Model file for the job. Use its own axes, mm. Face numbers are marked on the shaded views. A direction names the side the tool comes from. Coordinates: 2 decimals unless noted, no trailing zeros. Write each loop counter-clockwise with the first axis right and the second up, starting at its lowest first coordinate (ties: lowest second). Pieces come first, ordered by that corner, then holes.
Q1. Which spindle directions (+Z, -Z, +X, -X, +Y, -Y) get a long thin tool onto all of the face, cutting with end or side? Do the marked faces 4, 5 and 6. Say none if no direction does.
Q2. Drill centre lines: probe 1 along Y at (x, z) = (7.5, 0) (3 decimals); probe 2 along X at (y, z) = (0.5, -3.75); probe 3 along X at (y, z) = (-4.75, -1.5). Where is each one in solid material? Low to high.
Q3. Pull direction Y, two halves, no side cores. Call the marked faces 1, 2 and 3: released by +Y, released by -Y, zero draft, split by the parting line, or undercut.
Q4. Pin check, flat tips, straight feed: P1, Ø1, axis at y = 0, z = 1, coming from the -X side; P2, Ø2, axis at x = -5, z = 4, coming from the -Y side; P3, Ø1.5, axis at x = -5.5, y = 0.5, coming from the +Z side; P4, Ø4, axis at x = 1.5, y = -2.5, coming from the -Z side. Stop position of each tip, or through.
Q5. Band-saw the part on C-C, the plane x = 4. Write the cut outline in (y, z) (3 decimals), plus the area to 3 significant figures.
Q6. Band-saw the part on B-B, the plane x = 0.5. Write the cut outline in (y, z) (1 decimal).
from build123d import *

# Parameters (mm, degrees)
F0_W     = 11.1125
F0_H     = 3.175
F5_DEPTH = 3.175
F6_SIZE  = 0.254
F7_SIZE  = 0.508


with BuildPart() as f1:
    # F0 (on Front) → F1 (revolve)
    with BuildSketch(Plane.XZ):
        Polygon((-1.5875, 0), (-1.5875, 4.7625), (-1.5875, 5.55625), (-7.14375, 5.55625), (-7.14375, 0), align=None)
    revolve(axis=Axis((2.778125, 0, 0), (1, 0, 0)))

    # F0 (on Front) → F2 (revolve)
    with BuildSketch(Plane.XZ):
        Polygon((1.5875, 3.175), (1.5875, 4.7625), (-1.5875, 4.7625), (-1.5875, 0), (1.5875, 0), align=None)
    revolve(axis=Axis((2.778125, 0, 0), (1, 0, 0)))

    # F0 (on Front) → F3 (revolve)
    with BuildSketch(Plane.XZ):
        with Locations((7.14375, 1.5875)):
            Rectangle(F0_W, F0_H)
    revolve(axis=Axis((2.778125, 0, 0), (1, 0, 0)))

    # F4 (on face) → F5 (cut)
    with BuildSketch(Plane(origin=(-7.14375, 0, 0), x_dir=(0, -1, 0), z_dir=(-1, 0, 0))):
        Polygon((1.833087, 0), (0.916544, 1.5875), (-0.916544, 1.5875), (-1.833087, 0), (-0.916544, -1.5875), (0.916544, -1.5875), align=None)
    extrude(amount=-F5_DEPTH, mode=Mode.SUBTRACT)

    # F6
    f6_edges = [f1.edges().sort_by_distance(p)[0] for p in [
        (-7.14375, 0, -5.55625),
    ]]
    chamfer(f6_edges, length=F6_SIZE)

    # F7
    f7_edges = [f1.edges().sort_by_distance(p)[0] for p in [
        (12.7, 0, -3.175),
    ]]
    chamfer(f7_edges, length=F7_SIZE)


solid = f1.part
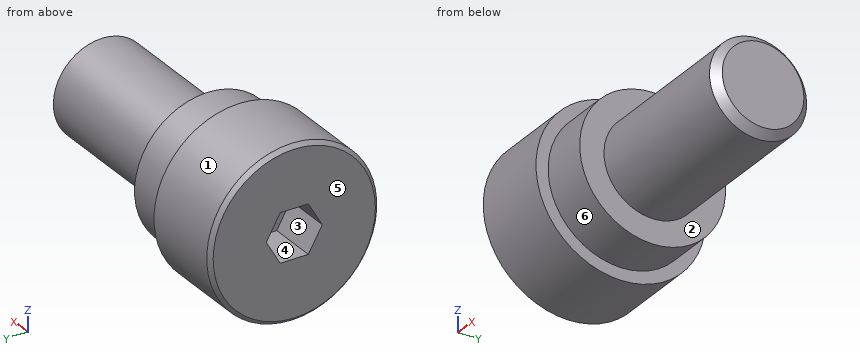
Answer sheet:
1. face 4: -X
1. face 5: +Z, -Z, -X, +Y, -Y
1. face 6: +X
2. probe 1: y = -3.175 to 3.175
2. probe 2: x = -7.14 to 1.59
2. probe 3: x = -7.14 to -1.59
3. face 1: split by the parting line
3. face 2: zero draft
3. face 3: undercut
4. P1: stops at x = -3.97
4. P2: stops at y = -4.68
4. P3: stops at z = 5.56
4. P4: stops at z = -4.74
5. outline: circle Ø6.35 at (0, 0)
5. area: 31.7 mm2
6. outline: circle Ø9.5 at (0, 0)
